Input: part model. Units: mm. Frame: model coordinates. A direction names the side the tool comes from. Coordinates: 2 decimals unless noted, no trailing zeros. Order: outer loops, then holes, each group sorted by start corner. A loop starts at its lowest first (then second) coordinate and runs counter-clockwise, first axis right, second up.
from build123d import *

# Parameters (mm, degrees)
SKETCH1_R           = 1.5
SKETCH1_R_2         = 10
BOSS_EXTRUDE1_DEPTH = 6.35


with BuildPart() as part:
    # Sketch1 → Boss-Extrude1 (new body)
    with BuildSketch(Plane(origin=(0, 0, 0), x_dir=(1, 0, 0), z_dir=(0, 1, 0))):
        Polygon((-25.5, 25.5), (-25.5, -25.5), (50.9, -25.5), (60.9, -25.5), (60.9, 6.061838244), (40.9, 6.061838244), (40.9, 16.061838244), (60.9, 16.061838244), (60.9, 25.5), align=None)
        with Locations((-15.5, 15.5)):
            Circle(SKETCH1_R, mode=Mode.SUBTRACT)
        with Locations((15.5, 15.5)):
            Circle(SKETCH1_R, mode=Mode.SUBTRACT)
        with Locations((15.5, -15.5)):
            Circle(SKETCH1_R, mode=Mode.SUBTRACT)
        with Locations((-15.5, -15.5)):
            Circle(SKETCH1_R, mode=Mode.SUBTRACT)
        Circle(SKETCH1_R_2, mode=Mode.SUBTRACT)
    extrude(amount=BOSS_EXTRUDE1_DEPTH)


solid = part.part
Item 1: Draft query along X for faces 1 (the face through (14, 3.13, -15.57)), 2 (the face through (17, 3, 25.5)), 3 (the face through (14, 3.13, 15.43)), 4 (the face through (60.9, 3, 10)). Return one class per face: pulls with the +X half, pulls with the -X half, needs draft (parallel to the pull), parting line crosses it, or undercut.
Response values:
face 1: undercut
face 2: needs draft
face 3: undercut
face 4: pulls with the +X half
Item 2: Cut plane C-C on x = 15.5. Return loops of the section in (y, z).
Response values:
outline: (0, -25.5) - (6.35, -25.5) - (6.35, -17) - (0, -17) - close; (0, -14) - (6.35, -14) - (6.35, 14) - (0, 14) - close; (0, 17) - (6.35, 17) - (6.35, 25.5) - (0, 25.5) - close
Item 3: Ray query, probe 1 along Z at (x, y) = (15.5, 4.25); probe 2 along X at (y, z) = (1.5, -15.5); probe 3 along Z at (x, y) = (55, 3.5). Return the intervals inside material, ascending.
Response values:
probe 1: z = -25.5 to -17, -14 to 14, 17 to 25.5
probe 2: x = -25.5 to -17, -14 to 14, 17 to 40.9
probe 3: z = -25.5 to -16.06, -6.06 to 25.5
Item 4: Cut plane A-A on z = 0. Return loops of the section in (x, y), then the cut area to 3 significant figures.
Response values:
outline: (-25.5, 0) - (-10, 0) - (-10, 6.35) - (-25.5, 6.35) - close; (10, 0) - (60.9, 0) - (60.9, 6.35) - (10, 6.35) - close
area: 422 mm2
Item 5: Access query for faces 5 (the face through (17, 6.35, 0)), 6 (the face through (51, 3, -16.062)). Directions: +Z, -Z, +X, -X, +Y, -Y. A direction counts if a zero-diameter tool reaches every point of the face in a straight line with its end or side. Return the directions, or none.
Response values:
face 5: +Z, -Z, +X, -X, +Y
face 6: +X, +Y, -Y
Item 6: Cut plane D-D on y = 4.5. Return loops of the section in (x, z), then the cut area to 3 significant figures.
Response values:
outline: (-25.5, -25.5) - (60.9, -25.5) - (60.9, -16.06) - (40.9, -16.06) - (40.9, -6.06) - (60.9, -6.06) - (60.9, 25.5) - (-25.5, 25.5) - close; hole circle Ø3 at (-15.5, -15.5); hole circle Ø3 at (-15.5, 15.5); hole circle Ø20 at (0, 0); hole circle Ø3 at (15.5, -15.5); hole circle Ø3 at (15.5, 15.5)
area: 3,860 mm2
Item 7: Cut plane B-B on x = 0. Return loops of the section in (y, z).
Response values:
outline: (0, -25.5) - (6.35, -25.5) - (6.35, -10) - (0, -10) - close; (0, 10) - (6.35, 10) - (6.35, 25.5) - (0, 25.5) - close
